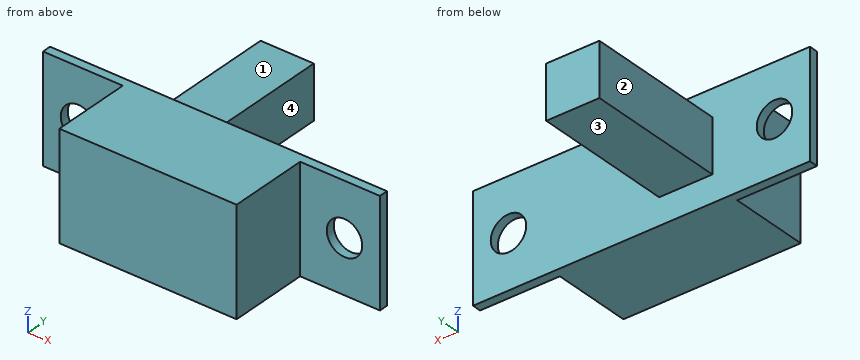
from build123d import *

# Parameters (mm, degrees)
SKETCH1_W           = 10
SKETCH1_H           = 6
BOSS_EXTRUDE1_DEPTH = 5
SKETCH2_W           = 19
SKETCH2_H           = 6
SKETCH2_R           = 1
BOSS_EXTRUDE2_DEPTH = 0.5
SKETCH3_W           = 3
SKETCH3_H           = 3
BOSS_EXTRUDE3_DEPTH = 8


with BuildPart() as part:
    # Sketch1 → Boss-Extrude1 (new body)
    with BuildSketch(Plane(origin=(0, 0, 0), x_dir=(1, 0, 0), z_dir=(0, 1, 0))):
        Rectangle(SKETCH1_W, SKETCH1_H)
    extrude(amount=BOSS_EXTRUDE1_DEPTH)

    # Sketch2 → Boss-Extrude2 (add)
    with BuildSketch(Plane(origin=(0, 5, 0), x_dir=(1, 0, 0), z_dir=(0, 1, 0))):
        Rectangle(SKETCH2_W, SKETCH2_H)
        with Locations(Location((-7.5, 0, 0), (0, 0, 270))):
            Circle(SKETCH2_R, mode=Mode.SUBTRACT)
        with Locations(Location((7.5, 0, 0), (0, 0, 270))):
            Circle(SKETCH2_R, mode=Mode.SUBTRACT)
    extrude(amount=-BOSS_EXTRUDE2_DEPTH)

    # Sketch3 → Boss-Extrude3 (add)
    with BuildSketch(Plane(origin=(0, 5, 0), x_dir=(1, 0, 0), z_dir=(0, 1, 0))):
        with Locations((-2.497009228, 0)):
            Rectangle(SKETCH3_W, SKETCH3_H)
    extrude(amount=BOSS_EXTRUDE3_DEPTH)


solid = part.part
CAD build for the part. Positions are in the model's coordinates, mm. Face numbers are marked on the shaded views. A direction names the side the tool comes from. Round coordinates to 2 decimals unless told otherwise and drop trailing zeros. Write each loop counter-clockwise with the first axis right and the second up, starting at its lowest first coordinate (ties: lowest second). Pieces come first, ordered by that corner, then holes. Notation, with made-up numbers: M 21,38.25 L 29,38.25 A23 cw 29,49.25 Z; hole C -33.5,41.25 d7. An arc over 180 degrees is marked long. Use a Markdown table: item, result. Add a question column.
1. Slice it at A-A on z = 0. Give the cut face in (x, y).
2. Slice it at D-D on y = 4.75. Give the cut face in (x, z).
3. 3-axis set-ups, long thin cutter, end or side, ignore diameter. For the marked faces 1, 2, 3 and 4: which of +Z, -Z, +X, -X, +Y, -Y reach the whole face in a straight line?
4. Slice it at B-B on x = 7.5. Give the cut face in (y, z), then the cut area to 3 significant figures.
5. Slice it at C-C on z = -2.5. Give the cut face in (x, y).
6. Flat gauge pins, fed straight in: P1, Ø0.9, axis at y = 9.5, z = 0, coming from the +X side; P2, Ø1.5, axis at y = 10.5, z = 2, coming from the -X side; P3, Ø2.5, axis at x = -2.5, y = 10.5, coming from the -Z side; P4, Ø6, axis at x = 1.5, y = 6, coming from the +Z side. Where does each tip first touch, or does it go through?
7. Drill centre lines: probe 1 along X at (y, z) = (4.6, 0); probe 2 along Z at (x, y) = (-1.5, 10.5); probe 3 along Y at (x, z) = (3, 1.55). Where is each one in solid material? Low to high.
Reply:
| question | item | result |
|---|---|---|
| 1 | outline | M -9.5,4.5 L -8.5,4.5 L -8.5,5 L -9.5,5 Z; M -6.5,4.5 L -5,4.5 L -5,0 L 5,0 L 5,4.5 L 6.5,4.5 L 6.5,5 L -1,5 L -1,13 L -4,13 L -4,5 L -6.5,5 Z; M 8.5,4.5 L 9.5,4.5 L 9.5,5 L 8.5,5 Z |
| 2 | outline | M -9.5,-3 L 9.5,-3 L 9.5,3 L -9.5,3 Z; hole C -7.5,0 d2; hole C 7.5,0 d2 |
| 3 | face 1 | +Z, +X, -X, +Y |
| 3 | face 2 | +Z, -Z, -X, +Y |
| 3 | face 3 | -Z, +X, -X, +Y |
| 3 | face 4 | +Z, -Z, +X, +Y |
| 4 | outline | M 4.5,-3 L 5,-3 L 5,-1 L 4.5,-1 Z; M 4.5,1 L 5,1 L 5,3 L 4.5,3 Z |
| 4 | area | 2.00 mm^2 |
| 5 | outline | M -9.5,4.5 L -5,4.5 L -5,0 L 5,0 L 5,4.5 L 9.5,4.5 L 9.5,5 L -9.5,5 Z |
| 6 | P1 | stops at x = -1 |
| 6 | P2 | stops at x = -4 |
| 6 | P3 | stops at z = -1.5 |
| 6 | P4 | stops at z = 3 |
| 7 | probe 1 | x = -9.5 to -8.5, -6.5 to 6.5, 8.5 to 9.5 |
| 7 | probe 2 | z = -1.5 to 1.5 |
| 7 | probe 3 | y = 0 to 5 |
